```python
from build123d import *

# Parameters (mm, degrees)
SKETCH_1_W      = 5
SKETCH_1_H      = 40
SKETCH_1_R      = 1.45
EXTRUDE_1_DEPTH = 27
SKETCH_2_W      = 120
SKETCH_2_H      = 5
SKETCH_2_R      = 1.45
EXTRUDE_2_DEPTH = 27


with BuildPart() as part:
    # 草图1 → 凸台-拉伸1 (new body)
    with BuildSketch(Plane(origin=(0, 0, 0), x_dir=(1, 0, 0), z_dir=(0, 1, 0))):
        Rectangle(SKETCH_1_W, SKETCH_1_H)
        with Locations(Location((0, 6, 0), (0, 0, 270))):
            Circle(SKETCH_1_R, mode=Mode.SUBTRACT)
        with Locations(Location((0, -10, 0), (0, 0, 270))):
            Circle(SKETCH_1_R, mode=Mode.SUBTRACT)
    extrude(amount=EXTRUDE_1_DEPTH)

    # 草图2 → 凸台-拉伸2 (add)
    with BuildSketch(Plane(origin=(0, 0, 0), x_dir=(1, 0, 0), z_dir=(0, 1, 0))):
        with Locations((-57.5, -19.5)):
            Rectangle(SKETCH_2_W, SKETCH_2_H)
        with Locations(Location((-10.04, -20, 0), (0, 0, 270))):
            Circle(SKETCH_2_R, mode=Mode.SUBTRACT)
        with Locations(Location((-103.24, -20, 0), (0, 0, 270))):
            Circle(SKETCH_2_R, mode=Mode.SUBTRACT)
    extrude(amount=EXTRUDE_2_DEPTH)


solid = part.part
```
Verification items for the finished model (mm, model axes). A direction names the side the tool comes from. Give positions to 0.01 mm unless a question says otherwise; leave off trailing zeros. Loops run counter-clockwise (first coordinate to the right, second up) from the corner with the lowest first, then second, coordinate; pieces in that order, holes last.
1. Go/stop test with flat-tipped pins: pin 1 Ø8 at (y, z) = (22.5, -13.5) entering from -X; pin 2 Ø6 at (x, y) = (-12, 7) entering from -Z. Record where each tip stops, or that it passes through.
2. Set-up check for faces 1 (the cylindrical face through (-104.526, 13.311, 20.669)), 2 (the flat face through (-61, 13, 17)): record each of +Z, -Z, +X, -X, +Y, -Y from which the full face is reachable in a straight line by a thin tool's end or side.
3. Section check B-B, the plane x = -103.24. Enter the section's corners in (y, z).
4. Thickness scan on line 1 (X direction, y = 14, z = 20); line 2 (X direction, y = 16.25, z = 10); line 3 (Z direction, x = -103.24, y = 11.5). Record the ranges inside material, lowest first.
5. Section check A-A, the plane z = 20. Enter the section's corners in (x, y).
6. Mould release check, pull along X, two halves, no side actions. Record for faces 3 (the flat face through (-2.5, 13, -1)), 4 (the cylindrical face through (0.06, 13.31, -7.45)), 5 (the flat face through (-49, 0, 18)): released by +X, released by -X, zero draft, split by the parting line, or undercut.
7. Section check C-C, the plane y = 22.5. Enter the section's corners in (x, z).
8. Section check D-D, the plane x = 0. Enter the section's corners in (y, z), then the cut area to 3 significant figures.
Geometry says:
1. pin 1: stops at x = -2.5
1. pin 2: stops at z = 17
2. face 1: +Y, -Y
2. face 2: -Z, -X, +Y, -Y
3. outline: (0, 17) - (27, 17) - (27, 18.55) - (0, 18.55) - close; (0, 21.45) - (27, 21.45) - (27, 22) - (0, 22) - close
4. line 1: x = -117.5 to -104.69, -101.79 to -11.49, -8.59 to 2.5
4. line 2: x = -2.5 to -1.45, 1.45 to 2.5
4. line 3: z = 17 to 18.55, 21.45 to 22
5. outline: (-117.5, 0) - (-104.69, 0) - (-104.69, 27) - (-117.5, 27) - close; (-101.79, 0) - (-11.49, 0) - (-11.49, 27) - (-101.79, 27) - close; (-8.59, 0) - (2.5, 0) - (2.5, 27) - (-8.59, 27) - close
6. face 3: released by -X
6. face 4: undercut
6. face 5: zero draft
7. outline: (-117.5, 17) - (-2.5, 17) - (-2.5, -20) - (2.5, -20) - (2.5, 22) - (-117.5, 22) - close; hole circle Ø2.9 at (-103.24, 20); hole circle Ø2.9 at (-10.04, 20); hole circle Ø2.9 at (0, -6); hole circle Ø2.9 at (0, 10)
8. outline: (0, -20) - (27, -20) - (27, -7.45) - (0, -7.45) - close; (0, -4.55) - (27, -4.55) - (27, 8.55) - (0, 8.55) - close; (0, 11.45) - (27, 11.45) - (27, 22) - (0, 22) - close
8. area: 977 mm2
